```python
from build123d import *

# Parameters (mm, degrees)
EXTRUDE_1_DEPTH     = 4
EXTRUDE_2_DEPTH     = 4
SKETCH_3_R          = 1.25
CUT_EXTRUDE_1_DEPTH = 15
CUT_EXTRUDE_2_DEPTH = 0.2


with BuildPart() as part:
    # 草图1 → 凸台-拉伸1 (new body)
    with BuildSketch(Plane(origin=(0, 0, 0), x_dir=(1, 0, 0), z_dir=(0, 1, 0))):
        with BuildLine():
            Line((-27.00005461, -31.987363475), (27.00005461, -31.987363475))
            ThreePointArc((27.00005461, -31.987363475), (29.112398272, -31.112402082), (29.987359665, -29.00005842))
            Line((29.987359665, -29.00005842), (29.987359665, 29.00005842))
            ThreePointArc((29.987359665, 29.00005842), (29.112398272, 31.112402082), (27.00005461, 31.987363475))
            Line((27.00005461, 31.987363475), (-27.00005461, 31.987363475))
            ThreePointArc((-27.00005461, 31.987363475), (-29.112398272, 31.112402082), (-29.987359665, 29.00005842))
            Line((-29.987359665, 29.00005842), (-29.987359665, -29.00005842))
            ThreePointArc((-29.987359665, -29.00005842), (-29.112398272, -31.112402082), (-27.00005461, -31.987363475))
        make_face()
    extrude(amount=EXTRUDE_1_DEPTH)

    # 草图2 → 凸台-拉伸2 (add)
    with BuildSketch(Plane.XZ):
        with BuildLine():
            Line((21.987359665, 23.987363475), (29.987359665, 23.987363475))
            Line((29.987359665, 23.987363475), (29.987359665, 29.00005842))
            ThreePointArc((29.987359665, 29.00005842), (29.112398272, 31.112402082), (27.00005461, 31.987363475))
            Line((27.00005461, 31.987363475), (21.987359665, 31.987363475))
            Line((21.987359665, 31.987363475), (21.987359665, 23.987363475))
        make_face()
        with BuildLine():
            Line((27.00005461, -31.987363475), (21.987359665, -31.987363475))
            Line((21.987359665, -31.987363475), (21.987359665, -23.987363475))
            Line((21.987359665, -23.987363475), (29.987359665, -23.987363475))
            Line((29.987359665, -23.987363475), (29.987359665, -29.00005842))
            ThreePointArc((29.987359665, -29.00005842), (29.112398272, -31.112402082), (27.00005461, -31.987363475))
        make_face()
        with BuildLine():
            Line((-21.987359665, 23.987363475), (-21.987359665, 31.987363475))
            Line((-21.987359665, 31.987363475), (-27.00005461, 31.987363475))
            ThreePointArc((-27.00005461, 31.987363475), (-29.112398272, 31.112402082), (-29.987359665, 29.00005842))
            Line((-29.987359665, 29.00005842), (-29.987359665, 23.987363475))
            Line((-29.987359665, 23.987363475), (-21.987359665, 23.987363475))
        make_face()
        with BuildLine():
            Line((-29.987359665, -23.987363475), (-29.987359665, -29.00005842))
            ThreePointArc((-29.987359665, -29.00005842), (-29.112398272, -31.112402082), (-27.00005461, -31.987363475))
            Line((-27.00005461, -31.987363475), (-21.987359665, -31.987363475))
            Line((-21.987359665, -31.987363475), (-21.987359665, -23.987363475))
            Line((-21.987359665, -23.987363475), (-29.987359665, -23.987363475))
        make_face()
    extrude(amount=EXTRUDE_2_DEPTH)

    # 草图3 → 切除-拉伸1 (cut)
    with BuildSketch(Plane.XZ.offset(4)):
        with Locations((-27.00005461, 29.00005842)):
            Circle(SKETCH_3_R)
        with Locations((27.00005461, 29.00005842)):
            Circle(SKETCH_3_R)
        with Locations((27.00005461, -29.00005842)):
            Circle(SKETCH_3_R)
        with Locations((-27.00005461, -29.00005842)):
            Circle(SKETCH_3_R)
    extrude(amount=-CUT_EXTRUDE_1_DEPTH, mode=Mode.SUBTRACT)

    # 草图5 → 切除-拉伸2 (cut)
    with BuildSketch(Plane(origin=(0, 4, 0), x_dir=(1, 0, 0), z_dir=(0, 1, 0))):
        with BuildLine():
            Line((-23, 25), (23, 25))
            ThreePointArc((23, 25), (24.414213562, 24.414213562), (25, 23))
            Line((25, 23), (25, -23))
            ThreePointArc((25, -23), (24.414213562, -24.414213562), (23, -25))
            Line((23, -25), (-23, -25))
            ThreePointArc((-23, -25), (-24.414213562, -24.414213562), (-25, -23))
            Line((-25, -23), (-25, 23))
            ThreePointArc((-25, 23), (-24.414213562, 24.414213562), (-23, 25))
        make_face()
        with BuildLine():
            Line((-20.309132479, 21.7161472), (11.083615015, 21.7161472))
            ThreePointArc((11.083615015, 21.7161472), (21.032992317, 9.959590783), (11.052213822, -1.770319196))
            Line((11.052213822, -1.770319196), (21.701392553, -13.464868734))
            Line((21.701392553, -13.464868734), (12.747815073, -13.464868734))
            Line((12.747815073, -13.464868734), (20.738271333, -22.160710638))
            Line((20.738271333, -22.160710638), (20.674664, -22.129263034))
            Line((20.674664, -22.129263034), (20.610679736, -22.097629074))
            Line((20.610679736, -22.097629074), (-2.958144095, -10.445151208))
            Line((-2.958144095, -10.445151208), (6.929882372, -10.445151208))
            Line((6.929882372, -10.445151208), (-0.976260078, -1.765140225))
            Line((-0.976260078, -1.765140225), (-6.216100572, -1.765140225))
            Line((-6.216100572, -1.765140225), (-9.975490326, -15.423548609))
            Line((-9.975490326, -15.423548609), (-9.977986633, -15.432618054))
            Line((-9.977986633, -15.432618054), (-22.608758584, -15.432618054))
            Line((-22.608758584, -15.432618054), (-20.552621384, -14.439759274))
            Line((-20.552621384, -14.439759274), (-14.742658641, 6.668678272))
            Line((-14.742658641, 6.668678272), (-8.710796679, 6.668678272))
            Line((-8.710796679, 6.668678272), (-14.742658641, 13.290950565))
            Line((-14.742658641, 13.290950565), (-20.309132479, 21.7161472))
        make_face(mode=Mode.SUBTRACT)
        with BuildLine():
            Line((3.367574747, 6.668678272), (-2.642308815, 13.268518768))
            Line((-2.642308815, 13.268518768), (9.694238704, 13.268518768))
            ThreePointArc((9.694238704, 13.268518768), (12.526480913, 9.96859852), (9.694238704, 6.668678272))
            Line((9.694238704, 6.668678272), (3.367574747, 6.668678272))
        make_face()
    extrude(amount=-CUT_EXTRUDE_2_DEPTH, mode=Mode.SUBTRACT)


solid = part.part
```
Geometry check sheet. Reference: the model listing, model coordinates, mm. A direction names the side the tool comes from. Give positions to 0.01 mm unless a question says otherwise; leave off trailing zeros. Order: outer loops, then holes, each group sorted by start corner. A loop starts at its lowest first (then second) coordinate and runs counter-clockwise, first axis right, second up. Notation, with made-up numbers: (63.5, 12.25) - (122.5, 12.25) arc R17 ccw to (122.5, 45.25) - close; hole circle Ø3 at (2, -32.5). An arc over 180 degrees is marked (long way). Answer in a Markdown table with one row per item. Add a question column.
Q1. Mould release check, pull along Z, two halves, no side actions. Record for faces 1 (the flat face through (0, 2, -31.987)), 2 (the flat face through (21.987, -2, 28)), 3 (the flat face through (26, -2, 23.987)): pulls with the +Z half, pulls with the -Z half, needs draft (parallel to the pull), parting line crosses it, or undercut.
Q2. Cross-section at A-A, the plane y = -2.5. Enter the section's corners in (x, z).
Q3. Material ranges on probe 1 along Z at (x, y) = (-25.5, -2); probe 2 along Z at (x, y) = (-26, 0.5); probe 3 along Y at (x, z) = (-5, -4), recorded low to high. Write a range as from..to.
Q4. Gauge pin test, flat ends, axial feed: pin 1 (1.5 mm diameter, centred on x = -6, z = -10, fed in from -Y); pin 2 (3 mm diameter, centred on y = -2, z = -3.5, fed in from +X). Record the tip position at first contact, or that the pin passes through.
Q5. Cross-section at B-B, the plane z = 27. Enter the section's corners in (x, y).
Q6. Cross-section at C-C, the plane x = 5. Enter the section's corners in (y, z), then the cut area to 3 significant figures.
Q7. Cross-section at D-D, the plane z = 7. Enter the section's corners in (x, y), then the cut area to 3 significant figures.
Q8. Tool access check on faces 4 (the flat face through (26, -4, -28)), 5 (the flat face through (7, 3.8, -10)), 6 (the flat face through (-21.987, -2, -28)), 7 (the flat face through (-26, -2, 23.987)). Record the directions out of +Z, -Z, +X, -X, +Y, -Y that give a thin tool (end or side, any length) a straight path to the whole face; none if there is none.
Check values:
| question | item | result |
|---|---|---|
| 1 | face 1 | pulls with the -Z half |
| 1 | face 2 | needs draft |
| 1 | face 3 | undercut |
| 2 | outline | (-29.99, -29) arc R2.99 ccw to (-27, -31.99) - (-21.99, -31.99) - (-21.99, -23.99) - (-29.99, -23.99) - close; (-29.99, 23.99) - (-21.99, 23.99) - (-21.99, 31.99) - (-27, 31.99) arc R2.99 ccw to (-29.99, 29) - close; (21.99, -31.99) - (27, -31.99) arc R2.99 ccw to (29.99, -29) - (29.99, -23.99) - (21.99, -23.99) - close; (21.99, 23.99) - (29.99, 23.99) - (29.99, 29) arc R2.99 ccw to (27, 31.99) - (21.99, 31.99) - close; hole circle Ø2.5 at (-27, -29); hole circle Ø2.5 at (-27, 29); hole circle Ø2.5 at (27, -29); hole circle Ø2.5 at (27, 29) |
| 3 | probe 1 | z = -31.99..-23.99, 23.99..31.99 |
| 3 | probe 2 | z = -31.99..-29.75, -28.25..28.25, 29.75..31.99 |
| 3 | probe 3 | y = 0..4 |
| 4 | pin 1 | stops at y = 0 |
| 4 | pin 2 | passes through |
| 5 | outline | (-29.99, -4) - (-21.99, -4) - (-21.99, 0) - (21.99, 0) - (21.99, -4) - (29.99, -4) - (29.99, 4) - (-29.99, 4) - close |
| 6 | outline | (0, -31.99) - (4, -31.99) - (4, -25) - (3.8, -25) - (3.8, -21.72) - (4, -21.72) - (4, -13.27) - (3.8, -13.27) - (3.8, -6.67) - (4, -6.67) - (4, 8.33) - (3.8, 8.33) - (3.8, 10.45) - (4, 10.45) - (4, 14.38) - (3.8, 14.38) - (3.8, 25) - (4, 25) - (4, 31.99) - (0, 31.99) - close |
| 6 | area | 251 mm^2 |
| 7 | outline | (-29.99, 0) - (29.99, 0) - (29.99, 4) - (25, 4) - (25, 3.8) - (15.81, 3.8) - (15.81, 4) - (3.79, 4) - (3.79, 3.8) - (-7.66, 3.8) - (-7.66, 4) - (-18.5, 4) - (-18.5, 3.8) - (-25, 3.8) - (-25, 4) - (-29.99, 4) - close |
| 7 | area | 234 mm^2 |
| 8 | face 4 | +Z, -Z, +X, -X, -Y |
| 8 | face 5 | +Y |
| 8 | face 6 | +Z, -Z, -Y |
| 8 | face 7 | +X, -X, -Y |
